Can you work these out from the model? Positions are in its coordinate system, mm. Face numbers are marked on the shaded views. A direction names the side the tool comes from. Give positions to 0.01 mm unless a question says otherwise; leave off trailing zeros. Order: outer loops, then holes, each group sorted by start corner. A loop starts at its lowest first (then second) coordinate and runs counter-clockwise, first axis right, second up. Notation, with made-up numbers: M 67,44 L 107,44 A15 cw 107,48 Z; hole C -20,81.25 d10. An arc over 180 degrees is marked long. Answer as a JSON object with one key per item and string values.
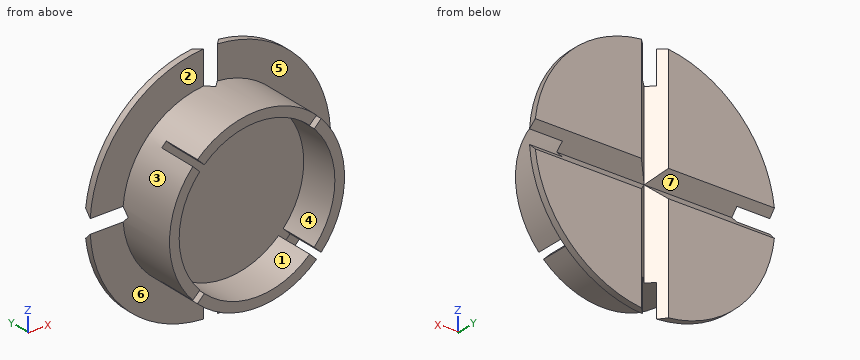
```python
from build123d import *

# Parameters (mm, degrees)
CUT_EXTRUDE1_DEPTH = 56.621758333
CIRPATTERN1_COUNT  = 4
SKETCH3_R          = 23.75
CUT_EXTRUDE2_DEPTH = 12
CUT_EXTRUDE3_START = 12
CUT_EXTRUDE3_DEPTH = 12
CIRPATTERN2_COUNT  = 4


with BuildPart() as part:
    # Sketch1 → Revolve1 (revolve)
    with BuildSketch(Plane(origin=(0, 0, 0), x_dir=(0, 0, -1), z_dir=(1, 0, 0)), mode=Mode.PRIVATE) as revolve1_sk:
        Polygon((0, 0), (26.7, 0), (26.7, 18), (36.7, 18), (36.7, 20), (0, 20), align=None)
    revolve(revolve1_sk.sketch.rotate(Axis((0, 20, 0), (0, -1, 0)), 180), axis=Axis((0, 20, 0), (0, -1, 0)))

    # Sketch2 → Cut-Extrude1 (cut, symmetric)
    with BuildSketch(Plane.XY):
        Polygon((4.121320344, 20), (0, 15.878679656), (-4.121320344, 20), align=None)
    cut_extrude1 = extrude(amount=CUT_EXTRUDE1_DEPTH, both=True, mode=Mode.SUBTRACT)

    # CirPattern1: Cut-Extrude1 ×4 about axis
    cirpattern1_axis = Axis((0, 0, 0), (0, 1, 0))
    for i in range(1, CIRPATTERN1_COUNT):
        add(cut_extrude1.rotate(cirpattern1_axis, i * 360 / CIRPATTERN1_COUNT), mode=Mode.SUBTRACT)

    # Sketch3 → Cut-Extrude2 (cut)
    with BuildSketch(Plane.XZ):
        with Locations(Location((0, 0, 0), (0, 0, 270))):
            Circle(SKETCH3_R)
    extrude(amount=-CUT_EXTRUDE2_DEPTH, mode=Mode.SUBTRACT)

    # Sketch4 → Cut-Extrude3 (cut)
    with BuildSketch(Plane(origin=(0, 0, 0), x_dir=(1, 0, 0), z_dir=(0, 1, 0)).offset(CUT_EXTRUDE3_START)):
        with BuildLine():
            Line((-25.234076692, -26.648290255), (0, -1.414213562))
            Line((0, -1.414213562), (-1.414213562, 0))
            Line((-1.414213562, 0), (-26.648290255, -25.234076692))
            ThreePointArc((-26.648290255, -25.234076692), (-25.95081887, -25.95081887), (-25.234076692, -26.648290255))
        make_face()
    cut_extrude3 = extrude(amount=-CUT_EXTRUDE3_DEPTH, mode=Mode.SUBTRACT)

    # CirPattern2: Cut-Extrude3 ×4 about axis
    cirpattern2_axis = Axis((0, 0, 0), (0, 1, 0))
    for i in range(1, CIRPATTERN2_COUNT):
        add(cut_extrude3.rotate(cirpattern2_axis, i * 360 / CIRPATTERN2_COUNT), mode=Mode.SUBTRACT)


solid = part.part
```
1) Thinking about a two-plate mould opening in Z: for the marked faces 1, 2 and 3, which applies, pulls with the +Z half, pulls with the -Z half, needs draft (parallel to the pull), parting line crosses it, or undercut?
Results found:
{"face 1": "undercut", "face 2": "needs draft", "face 3": "parting line crosses it"}
2) I want a section at C-C on z = -21. Write out the boundary of the cut face in (x, y), and give its area (3 significant figures).
Results found:
{"outline": "M -30.1,18 L -16.49,18 L -16.49,0 L -11.09,0 L -11.09,12 L 11.09,12 L 11.09,0 L 16.49,0 L 16.49,18 L 30.1,18 L 30.1,20 L 4.12,20 L 0,15.88 L -4.12,20 L -30.1,20 Z", "area": "431 mm²"}
3) For the marked faces 4, 5, 6 and 7, which set-ups out of +Z, -Z, +X, -X, +Y, -Y let a thin tool reach every point of the face, with its end or its side?
Results found:
{"face 4": "-Y", "face 5": "+Z, +X, -Y", "face 6": "-Z, -X, -Y", "face 7": "+X, -X, +Y"}
4) I need wall thicknesses on L1, parallel to X at y = 4.75, z = 0.5; L2, parallel to Z at x = 16, y = 4.25; L3, parallel to Y at x = 14, z = 15. Which ranges of each line are inside material? Lowest first, please.
Results found:
{"L1": "x = -26.7 to -23.74, 23.74 to 26.7", "L2": "z = -21.37 to -17.55, 17.55 to 21.37", "L3": "y = 12 to 20"}
5) I want a section at A-A on z = 30.5. Write out the boundary of the cut face in (x, y), and give its area (3 significant figures).
Results found:
{"outline": "M -20.41,18 L -2.12,18 L -4.12,20 L -20.41,20 Z; M 2.12,18 L 20.41,18 L 20.41,20 L 4.12,20 Z", "area": "69.2 mm²"}
6) I want a section at B-B on z = -8. Write out the boundary of the cut face in (x, y).
Results found:
{"outline": "M -35.82,18 L -25.47,18 L -25.47,0 L -22.36,0 L -22.36,12 L 22.36,12 L 22.36,0 L 25.47,0 L 25.47,18 L 35.82,18 L 35.82,20 L 4.12,20 L 0,15.88 L -4.12,20 L -35.82,20 Z"}
7) I'm going to push flat-ended pins straight in: pin 1 Ø8 at (x, y) = (8.5, 11.5) entering from -Z; pin 2 Ø12 at (x, y) = (10.5, 17.5) entering from -Z; pin 3 Ø12 at (y, z) = (4.5, -11) entering from +X. Where does each tip first touch, or does it pass through?
Results found:
{"pin 1": "stops at z = -26.32", "pin 2": "stops at z = -36.42", "pin 3": "stops at x = 26.23"}
